from build123d import *

# Parameters (mm, degrees)
F0_W     = 50.8
F0_H     = 76.2
F0_W_2   = 44.45
F0_H_2   = 69.85
F2_DEPTH = 152.4
F3_R     = 3.175


# Not quite as in the source:
# - a variable given as a bare number and used for a length is read in inches; the dataset says mm whatever the document's units were


with BuildPart() as f2:
    # F0 (on Top) → F2 (new body)
    with BuildSketch(Plane.XY):
        Rectangle(F0_W, F0_H)
        Rectangle(F0_W_2, F0_H_2, mode=Mode.SUBTRACT)
    extrude(amount=F2_DEPTH)

    # F3
    f3_edges = [f2.edges().sort_by_distance(p)[0] for p in [
        (-22.225, 34.925, 76.2),
        (22.225, 34.925, 76.2),
        (22.225, -34.925, 76.2),
        (-22.225, -34.925, 76.2),
        (25.4, 38.1, 76.2),
        (-25.4, 38.1, 76.2),
        (25.4, -38.1, 76.2),
        (-25.4, -38.1, 76.2),
    ]]
    fillet(f3_edges, radius=F3_R)


solid = f2.part
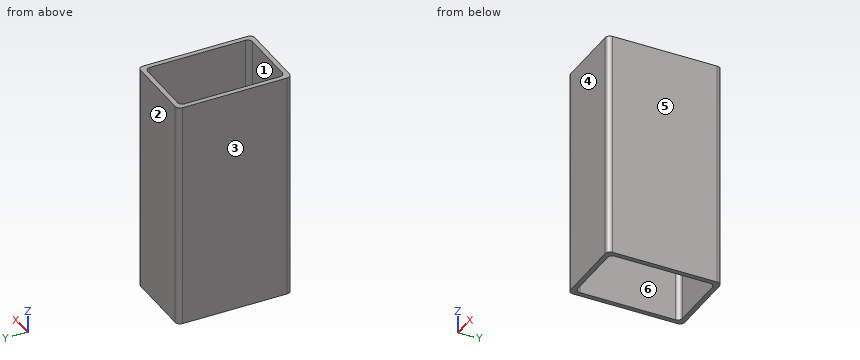
Can you work these out from the model? Positions are in its coordinate system, mm. Face numbers are marked on the shaded views. A direction names the side the tool comes from. Coordinates: 2 decimals unless noted, no trailing zeros. Loops run counter-clockwise (first coordinate to the right, second up) from the corner with the lowest first, then second, coordinate; pieces in that order, holes last. Notation, with made-up numbers: (86, 36) - (102, 36) arc R27 cw to (102, 73) - close; hole circle Ø11 at (16, 80). An arc over 180 degrees is marked (long way). Answer as a JSON object with one key per item and string values. Group by question number.
Item 1: If we section it at A-A (x = 13): List the corners of the cut face in (y, z) for me (3 decimals), plus the area to 3 significant figures.
Item 2: On a 3-axis mill with a long thin cutter (end or side, diameter ignored), from which of +Z, -Z, +X, -X, +Y, -Y can I reach the whole of each face in a straight line? I mean the marked faces 5 and 6. Say none if no direction works.
Item 3: If I drill on L1, parallel to Y at x = -18.5, z = 31.5 (3 decimals); L2, parallel to X at y = -7.5, z = 26 (3 decimals); L3, parallel to Y at x = 21, z = 140.5, over which ranges is the centre line in solid material (lowest first)? Write a range as from..to.
Item 4: If we mould it in two halves opening along Y, with no side actions, what happens to the marked faces 1, 2, 3 and 4? For each: released by +Y, released by -Y, zero draft, split by the parting line, or undercut.
Item 5: If we section it at B-B (y = 26): List the corners of the cut face in (x, z) for me (3 decimals), plus the area to 3 significant figures.
Item 6: If we section it at C-C (z = 30): List the corners of the cut face in (x, y) for me (3 decimals).
Returned:
{
 "1": {"outline": "(-38.1, 0) - (-34.925, 0) - (-34.925, 152.4) - (-38.1, 152.4) - close; (34.925, 0) - (38.1, 0) - (38.1, 152.4) - (34.925, 152.4) - close", "area": "968 mm²"},
 "2": {"face 5": "+Z, -Z, +X, +Y, -Y", "face 6": "+Z, -Z"},
 "3": {"L1": "y = -38.1..-34.925, 34.925..38.1", "L2": "x = -25.4..-22.225, 22.225..25.4", "L3": "y = -38.1..-34.26, 34.26..38.1"},
 "4": {"face 1": "undercut", "face 2": "released by +Y", "face 3": "zero draft", "face 4": "released by -Y"},
 "5": {"outline": "(-25.4, 0) - (-22.225, 0) - (-22.225, 152.4) - (-25.4, 152.4) - close; (22.225, 0) - (25.4, 0) - (25.4, 152.4) - (22.225, 152.4) - close", "area": "968 mm²"},
 "6": {"outline": "(-25.4, -34.925) arc R3.175 ccw to (-22.225, -38.1) - (22.225, -38.1) arc R3.175 ccw to (25.4, -34.925) - (25.4, 34.925) arc R3.175 ccw to (22.225, 38.1) - (-22.225, 38.1) arc R3.175 ccw to (-25.4, 34.925) - close; hole (-22.225, -31.75) arc R3.175 ccw to (-19.05, -34.925) - (19.05, -34.925) arc R3.175 ccw to (22.225, -31.75) - (22.225, 31.75) arc R3.175 ccw to (19.05, 34.925) - (-19.05, 34.925) arc R3.175 ccw to (-22.225, 31.75) - close"}
}
